```python
from build123d import *

# Parameters (mm, degrees)
F0_R     = 12.5
F1_DEPTH = 4


with BuildPart() as f1:
    # F0 (on Top) → F1 (new body)
    with BuildSketch(Plane.XY):
        Circle(F0_R)
        with BuildLine():
            ThreePointArc((8.672397, -5.323291), (0, -10.175849), (-8.672397, -5.323291))
            Line((-8.672397, -5.323291), (0, -3.602296))
            Line((0, -3.602296), (8.672397, -5.323291))
        make_face(mode=Mode.SUBTRACT)
        with BuildLine():
            ThreePointArc((-8.946304, -4.848871), (-8.812543, 5.087924), (-0.273907, 10.172161))
            Line((-0.273907, 10.172161), (-3.11968, 1.801148))
            Line((-3.11968, 1.801148), (-8.946304, -4.848871))
        make_face(mode=Mode.SUBTRACT)
        with BuildLine():
            Line((3.11968, 1.801148), (0.273907, 10.172161))
            ThreePointArc((0.273907, 10.172161), (8.812543, 5.087924), (8.946304, -4.848871))
            Line((8.946304, -4.848871), (3.11968, 1.801148))
        make_face(mode=Mode.SUBTRACT)
    extrude(amount=F1_DEPTH)

    # F2 (on Front) → F3 (revolve)
    with BuildSketch(Plane.XZ):
        Polygon((-1.25, 5.5), (-1.25, 3.62873), (0, 2.650845), (0, 6), (-1.503677, 6), align=None)
    revolve(axis=Axis((0, 0, 4.325422), (0, 0, -1)))


solid = f1.part
```
Can you work these out from the model? Positions are in its coordinate system, mm. Coordinates: 2 decimals unless noted, no trailing zeros. Loops run counter-clockwise (first coordinate to the right, second up) from the corner with the lowest first, then second, coordinate; pieces in that order, holes last.
Item 1: Suppose I cut it at C-C (x = -4.75). Please give me the cut outline in (y, z).
Answers below:
outline: (-11.56, 0) - (-9, 0) - (-9, 4) - (-11.56, 4) - close; (-4.54, 0) - (-0.06, 0) - (-0.06, 4) - (-4.54, 4) - close; (9, 0) - (11.56, 0) - (11.56, 4) - (9, 4) - close
Item 2: If we mould it in two halves opening along Z, with no side actions, what happens to faces 1 (the face through (0, 0, 6)), 2 (the face through (-5.992, -1.477, 1.972)), 3 (the face through (0, 0, 0)), 4 (the face through (0.27, -1.22, 4.74))? For each: released by +Z, released by -Z, zero draft, split by the parting line, or undercut.
Answers below:
face 1: released by +Z
face 2: zero draft
face 3: released by -Z
face 4: undercut
Item 3: Please list where these lines run through material, in increasing order: L1, parallel to Y at x = -5.25, z = 3.5; L2, parallel to X at y = 7, z = 0.55; L3, parallel to X at y = -0.75, z = 0.9.
Answers below:
L1: y = -11.34 to -8.72, -4.64 to -0.63, 8.72 to 11.34
L2: x = -10.36 to -7.39, -1.35 to 1.35, 7.39 to 10.36
L3: x = -12.48 to -10.15, -5.35 to 5.35, 10.15 to 12.48
Item 4: Suppose I cut it at B-B (y = 6.25). Please give me the cut outline in (x, z), then the cut area to 3 significant figures.
Answers below:
outline: (-10.83, 0) - (-8.03, 0) - (-8.03, 4) - (-10.83, 4) - close; (-1.61, 0) - (1.61, 0) - (1.61, 4) - (-1.61, 4) - close; (8.03, 0) - (10.83, 0) - (10.83, 4) - (8.03, 4) - close
area: 35.2 mm2
Item 5: Suppose I cut it at A-A (z = 0.85). Please give me the cut outline in (x, y).
Answers below:
outline: circle Ø25 at (0, 0); hole (-8.95, -4.85) - (-3.12, 1.8) - (-0.27, 10.17) arc R10.18 ccw to start; hole (-8.67, -5.32) arc R10.18 ccw to (8.67, -5.32) - (0, -3.6) - close; hole (0.27, 10.17) - (3.12, 1.8) - (8.95, -4.85) arc R10.18 ccw to start
Item 6: I'm going to push flat-ended pins straight in: pin 1 (3 mm diameter, centred on x = 1.5, y = 8, fed in from +Z); pin 2 (1 mm diameter, centred on x = 4.5, z = 3, fed in from -Y); pin 3 (3 mm diameter, centred on x = -6.5, z = 1, fed in from +Y). Where does each tip first touch, or does it pass through?
Answers below:
pin 1: stops at z = 4
pin 2: stops at y = -11.84
pin 3: stops at y = 11.46
Item 7: Suppose I cut it at D-D (y = -7.5). Please give me the cut outline in (x, z).
Answers below:
outline: (-10, 0) - (-6.88, 0) - (-6.88, 4) - (-10, 4) - close; (6.88, 0) - (10, 0) - (10, 4) - (6.88, 4) - close
